Geometry: final body of the model. Coordinates: model frame, mm. Give positions to 0.01 mm unless a question says otherwise; leave off trailing zeros. Write each loop counter-clockwise with the first axis right and the second up, starting at its lowest first coordinate (ties: lowest second). Pieces come first, ordered by that corner, then holes. Notation, with made-up numbers: M 76,-38.5 L 92,-38.5 A19 cw 92,-28.5 Z; hole C 16,68.5 d1. An arc over 180 degrees is marked long. Answer as a JSON object with one key per item and string values.
from build123d import *

# Parameters (mm, degrees)
SKETCH1_R           = 13.97
BOSS_EXTRUDE1_DEPTH = 5.08


with BuildPart() as part:
    # Sketch1 → Boss-Extrude1 (new body)
    with BuildSketch(Plane(origin=(0, 0, 0), x_dir=(1, 0, 0), z_dir=(0, 1, 0))):
        with Locations(Location((0, 0, 0), (0, 0, 270))):
            Circle(SKETCH1_R)
    extrude(amount=BOSS_EXTRUDE1_DEPTH)

    # Sketch5 → Cut-Revolve3 (revolve, cut)
    with BuildSketch(Plane(origin=(7.9502, 0, 0), x_dir=(0, 0, -1), z_dir=(1, 0, 0))):
        with BuildLine():
            Line((0, 5.08), (0, 2.0955))
            ThreePointArc((0, 2.0955), (-2.110360188, 2.969639812), (-2.9845, 5.08))
            Line((-2.9845, 5.08), (0, 5.08))
        make_face()
    cut_revolve3 = revolve(axis=Axis((7.9502, 5.08, 0), (0, -1, 0)), mode=Mode.SUBTRACT)

    # Mirror3: Cut-Revolve3 across plane
    add(cut_revolve3.mirror(Plane(origin=(0, 0, 0), x_dir=(0, 0, 1), z_dir=(1, 0, 0))), mode=Mode.SUBTRACT)

    # Sketch3 → Cut-Revolve4 (revolve, cut)
    with BuildSketch(Plane.XY.offset(-9.271)):
        with BuildLine():
            Line((0, 5.08), (0, 2.0955))
            ThreePointArc((0, 2.0955), (2.110360188, 2.969639812), (2.9845, 5.08))
            Line((2.9845, 5.08), (0, 5.08))
        make_face()
    cut_revolve4 = revolve(axis=Axis((0, 5.08, -9.271), (0, -1, 0)), mode=Mode.SUBTRACT)

    # Mirror4: Cut-Revolve4 across plane
    add(cut_revolve4.mirror(Plane.XY), mode=Mode.SUBTRACT)


solid = part.part
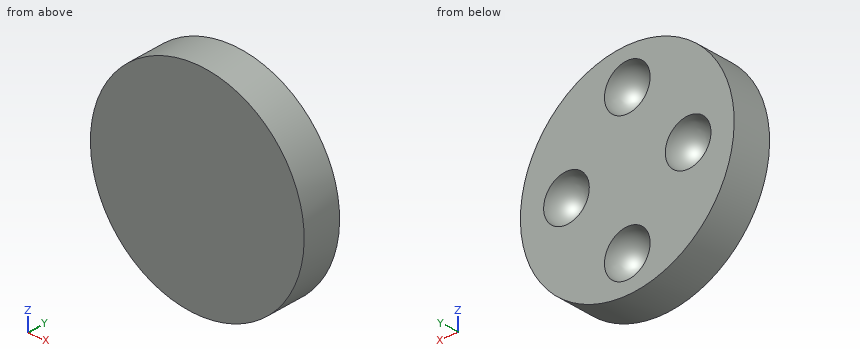
1) Cut plane A-A on x = 0. Return loops of the section in (y, z), and give its area (3 significant figures).
Geometry check:
{"outline": "M 0,-13.97 L 5.08,-13.97 L 5.08,-12.26 A2.98 cw 5.08,-6.29 L 5.08,6.29 A2.98 cw 5.08,12.26 L 5.08,13.97 L 0,13.97 Z", "area": "114 mm2"}
2) Cut plane D-D on y = 0.9. Return loops of the section in (x, z), and give its area (3 significant figures).
Geometry check:
{"outline": "C 0,0 d27.94", "area": "613 mm2"}
3) Cut plane B-B on y = 2.7. Return loops of the section in (x, z), and give its area (3 significant figures).
Geometry check:
{"outline": "C 0,0 d27.94; hole C -7.95,0 d3.6; hole C 0,-9.27 d3.6; hole C 0,9.27 d3.6; hole C 7.95,0 d3.6", "area": "572 mm2"}
4) Cut plane C-C on z = 0. Return loops of the section in (x, y), and give its area (3 significant figures).
Geometry check:
{"outline": "M -13.97,0 L 13.97,0 L 13.97,5.08 L 10.93,5.08 A2.98 cw 4.97,5.08 L -4.97,5.08 A2.98 cw -10.93,5.08 L -13.97,5.08 Z", "area": "114 mm2"}
5) Contact query for flat-ended pins moving along their axis: P1, Ø2, axis at y = 1.5, z = -10.5, coming from the -X side; P2, Ø2, axis at y = 1.5, z = -8, coming from the +X side; P3, Ø1.5, axis at y = 3.5, z = 7, coming from the -X side. Output: stop coordinate, or through.
Geometry check:
{"P1": "stops at x = -10.24", "P2": "stops at x = 12.09", "P3": "stops at x = -12.49"}
6) Line query: line 1 (X direction, y = 4.45, z = -1); line 2 (Z direction, x = -0.75, y = 3.75); line 3 (X direction, y = 4.15, z = -11). Output: solid intervals per line, ascending. Write a range as from..to.
Geometry check:
{"line 1": "x = -13.93..-10.69, -5.21..5.21, 10.69..13.93", "line 2": "z = -13.95..-11.84, -6.71..6.71, 11.84..13.95", "line 3": "x = -8.61..-2.25, 2.25..8.61"}
